Could you check a few things on this model? Use its own coordinates, in mm. Coordinates: 2 decimals unless noted, no trailing zeros. Loops run counter-clockwise (first coordinate to the right, second up) from the corner with the lowest first, then second, coordinate; pieces in that order, holes last. Notation, with made-up numbers: (29, 30.25) - (77, 30.25) arc R28 ccw to (77, 54.25) - close; hole circle Ø6 at (73.25, 49.25). An arc over 180 degrees is marked (long way). One line per question, with ' | ' between items. Start each with the question number.
1. I'm going to push flat-ended pins straight in: P1, Ø3.5, axis at y = 10.86, z = -385, coming from the +X side; P2, Ø6, axis at x = -4.5, z = -293, coming from the +Y side; P3, Ø2, axis at x = 8, y = 42.5, coming from the -Z side; P4, Ø6, axis at x = -3, z = -386, coming from the +Y side. Where does each tip first touch, or does it pass through?
2. I want a section at A-A, the plane y = 0. Write out the boundary of the cut face in (x, z).
3. Please list where these lines run through material, in increasing order: L1, parallel to Z at x = -20, y = 54.5; L2, parallel to Z at x = 8, y = -51; L3, parallel to Y at x = 3, z = -65.5. Write a range as [from, to].
4. I want a section at D-D, the plane y = -46.5. Write out the boundary of the cut face in (x, z).
5. I want a section at C-C, the plane z = -256. Write out the boundary of the cut face in (x, y).
6. I want a section at B-B, the plane x = 0. Write out the boundary of the cut face in (y, z), then the cut area to 4 significant figures.
from build123d import *

# Parameters (mm, degrees)
BOSS_EXTRU_1_DEPTH      = 5
BOSS_EXTRU_3_DEPTH      = 20
ESQUISSE7_R             = 3
ENL_V_MAT_EXTRU_1_DEPTH = 20


with BuildPart() as part:
    # Esquisse1 → Boss.-Extru.1 (new body)
    with BuildSketch(Plane.XY):
        with BuildLine():
            Line((-10, -74.330343737), (-10, -94.330343737))
            Line((-10, -94.330343737), (10, -94.330343737))
            Line((10, -94.330343737), (10, -74.330343737))
            ThreePointArc((10, -74.330343737), (0, 75), (-10, -74.330343737))
        make_face()
    extrude(amount=BOSS_EXTRU_1_DEPTH)

    # Esquisse6 → Boss.-Extru.3 (add)
    with BuildSketch(Plane(origin=(10, 0, 0), x_dir=(0, 0, -1), z_dir=(1, 0, 0))):
        Polygon((375, -20), (320.669656263, -74.330343737), (-5, -74.330343737), (-5, -94.330343737), (328.953927511, -94.330343737), (395, -28.284271247), (395, 20), (375, 20), align=None)
    extrude(amount=-BOSS_EXTRU_3_DEPTH)

    # Esquisse7 → Enlèv. mat.-Extru.1 (cut)
    with BuildSketch(Plane(origin=(10, 0, 0), x_dir=(0, 0, -1), z_dir=(1, 0, 0))):
        with Locations(Location((324.811791887, -84.330343737, 0), (0, 0, 90))):
            Circle(ESQUISSE7_R)
        with Locations(Location((385, -24.142135624, 0), (0, 0, 90))):
            Circle(ESQUISSE7_R)
        with Locations(Location((385, 10.857864376, 0), (0, 0, 90))):
            Circle(ESQUISSE7_R)
        with Locations(Location((25, -84.330343737, 0), (0, 0, 90))):
            Circle(ESQUISSE7_R)
    extrude(amount=-ENL_V_MAT_EXTRU_1_DEPTH, mode=Mode.SUBTRACT)


solid = part.part
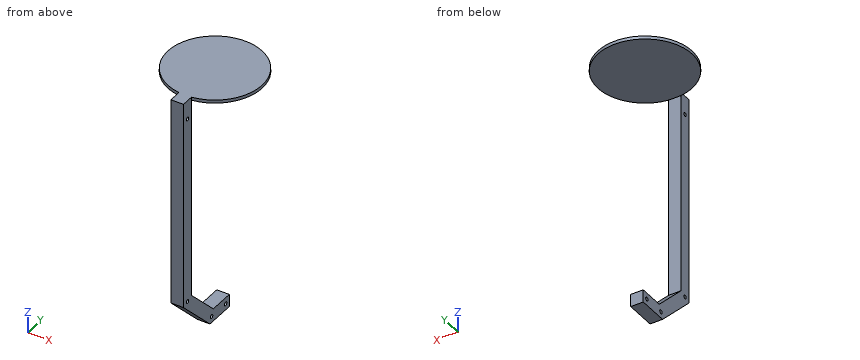
Results are:
1) P1: passes through | P2: stops at y = -74.33 | P3: stops at z = 0 | P4: stops at y = 20
2) outline: (-75, 0) - (75, 0) - (75, 5) - (-75, 5) - close; (-10, -395) - (10, -395) - (10, -375) - (-10, -375) - close
3) L1: z = [0, 5] | L2: z = [-372.28, -344], [0, 5] | L3: y = [-94.33, -74.33]
4) outline: (-58.85, 0) - (58.85, 0) - (58.85, 5) - (-58.85, 5) - close; (-10, -376.78) - (10, -376.78) - (10, -348.5) - (-10, -348.5) - close
5) outline: (-10, -94.33) - (10, -94.33) - (10, -74.33) - (-10, -74.33) - close
6) outline: (-94.33, -328.95) - (-28.28, -395) - (20, -395) - (20, -375) - (-20, -375) - (-74.33, -320.67) - (-74.33, 0) - (75, 0) - (75, 5) - (-94.33, 5) - close; hole circle Ø6 at (-84.33, -324.81); hole circle Ø6 at (-84.33, -25); hole circle Ø6 at (-24.14, -385); hole circle Ø6 at (10.86, -385) | area: 9,815 mm2
